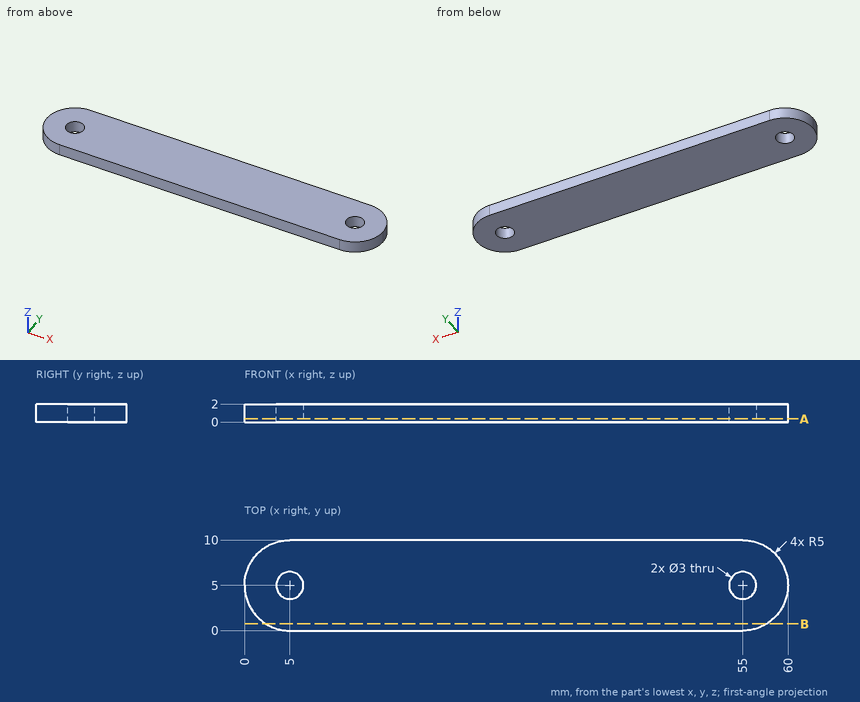
Study the drawing (mm; zero at the part's minimum x, y, z) and answer. Round coordinates to 2 decimals unless told otherwise and drop trailing zeros. Write each loop counter-clockwise with the first axis right and the second up, starting at its lowest first coordinate (ties: lowest second). Pieces come first, ordered by that corner, then holes. Notation, with made-up numbers: (-34.5, 86.5) -> (6.5, 86.5) arc R20 ccw to (6.5, 118.5) -> close; hole circle Ø3 at (37.25, 89). An arc over 180 degrees is marked (long way). Answer as CSV lines item,"result". Start each with the question number.
(1) Find the intervals of material crossed by probe 1 along X at (y, z) = (6.25, 1.6); probe 2 along X at (y, z) = (5.75, 0.95); probe 3 along Y at (x, z) = (55, 1.4), in increasing order.
(2) The part is cut by section A-A, the plane z = 0.35. Give the number of separate pieces and of enclosed holes in the cut face, then the cut area to 3 significant figures.
(3) The part is cut by section B-B, the plane y = 0.75. Give the vertices of the cut face in (x, z).
Output values:
1,probe 1,"x = 0.16 to 4.17, 5.83 to 54.17, 55.83 to 59.84"
1,probe 2,"x = 0.06 to 3.7, 6.3 to 53.7, 56.3 to 59.94"
1,probe 3,"y = 0 to 3.5, 6.5 to 10"
2,separate pieces,"1"
2,enclosed holes,"2"
2,area,"564 mm²"
3,outline,"(2.37, 0) -> (57.63, 0) -> (57.63, 2) -> (2.37, 2) -> close"
